Here's how the part is built. I have some questions about the finished solid (model axes, mm). Face numbers are marked on the shaded views. A direction names the side the tool comes from. Give positions to 0.01 mm unless a question says otherwise; leave off trailing zeros. Order: outer loops, then holes, each group sorted by start corner. A loop starts at its lowest first (then second) coordinate and runs counter-clockwise, first axis right, second up. Notation, with made-up numbers: M 29,66.25 L 35,66.25 A13 ccw 35,91.25 Z; hole C -21.75,8 d1. An arc over 180 degrees is marked long. One line per item, written item: value. Start each with the question number.
from build123d import *

# Parameters (mm, degrees)
F0_W     = 38.1
F0_H     = 50.8
F1_DEPTH = 12.7
F2_R     = 1.65
F2_R_2   = 3.5
F3_DEPTH = 12.701
F4_W     = 10
F4_H     = 5
F5_DEPTH = 50.801


with BuildPart() as f1:
    # F0 (on Top) → F1 (new body)
    with BuildSketch(Plane.XY):
        with Locations((19.05, 25.4)):
            Rectangle(F0_W, F0_H)
    extrude(amount=F1_DEPTH)

    # F2 (on face) → F3 (cut, through all)
    with BuildSketch(Plane.XY.offset(12.7)):
        with Locations((8.25, 5)):
            Circle(F2_R)
        with Locations((29.85, 5)):
            Circle(F2_R)
        with Locations((8.25, 25.35)):
            Circle(F2_R)
        with Locations((19.05, 43.5)):
            Circle(F2_R_2)
    extrude(amount=-F3_DEPTH, mode=Mode.SUBTRACT)

    # F4 (on face) → F5 (cut, through all)
    with BuildSketch(Plane.XZ):
        with Locations((18.962298, 2.5)):
            Rectangle(F4_W, F4_H)
    extrude(amount=-F5_DEPTH, mode=Mode.SUBTRACT)


solid = f1.part
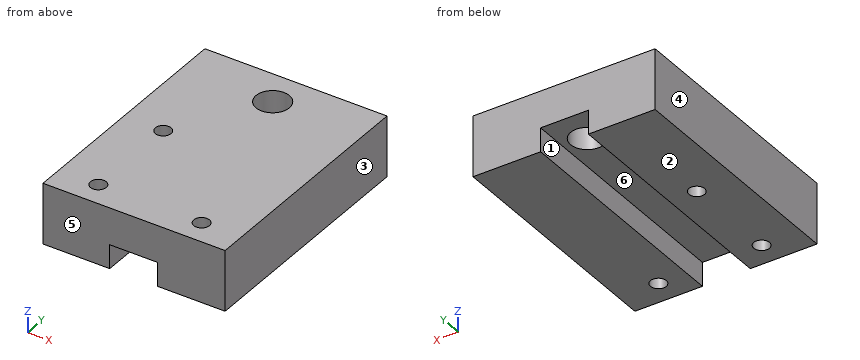
Item 1: Will these pins go through, and if not, where does the flat tip stop? P1, Ø8, axis at x = 19.5, y = 32, coming from the -Z side; P2, Ø2, axis at x = 8.25, y = 25.35, coming from the +Z side.
Item 2: I want a section at D-D on x = 19.05. Write out the boundary of the cut face in (y, z), plus the area to 3 significant figures.
Item 3: I want a section at C-C on y = 43.5. Write out the boundary of the cut face in (x, z).
Item 4: For the marked faces 5 and 6, which set-ups out of +Z, -Z, +X, -X, +Y, -Y let a thin tool reach every point of the face, with its end or its side?
Item 5: We'd pull the mould along X, two halves only. Please class the marked faces 1, 2, 3 and 4: +X half, -X half, draft (parallel to the pull), parting line (faces both ways), or undercut.
Item 6: Please list where these lines run through material, in increasing order: probe 1 along Y at (x, z) = (8.25, 8.5); probe 2 along Y at (x, z) = (19.05, 10); probe 3 along X at (y, z) = (20, 2.75). Write a range as [from, to].
Item 7: I want a section at A-A on z = 4. Write out the boundary of the cut face in (x, y), plus the area to 3 significant figures.
Item 8: I want a section at B-B on x = 8.25. Write out the boundary of the cut face in (y, z), plus the area to 3 significant figures.
Answer below:
1. P1: stops at z = 5
1. P2: passes through
2. outline: M 0,5 L 40,5 L 40,12.7 L 0,12.7 Z; M 47,5 L 50.8,5 L 50.8,12.7 L 47,12.7 Z
2. area: 337 mm²
3. outline: M 0,0 L 13.96,0 L 13.96,5 L 15.55,5 L 15.55,12.7 L 0,12.7 Z; M 22.55,5 L 23.96,5 L 23.96,0 L 38.1,0 L 38.1,12.7 L 22.55,12.7 Z
4. face 5: +Z, -Z, +X, -X, -Y
4. face 6: -Z, +Y, -Y
5. face 1: undercut
5. face 2: draft
5. face 3: +X half
5. face 4: -X half
6. probe 1: y = [0, 3.35], [6.65, 23.7], [27, 50.8]
6. probe 2: y = [0, 40], [47, 50.8]
6. probe 3: x = [0, 13.96], [23.96, 38.1]
7. outline: M 0,0 L 13.96,0 L 13.96,50.8 L 0,50.8 Z; M 23.96,0 L 38.1,0 L 38.1,50.8 L 23.96,50.8 Z; hole C 8.25,5 d3.3; hole C 8.25,25.35 d3.3; hole C 29.85,5 d3.3
7. area: 1,400 mm²
8. outline: M 0,0 L 3.35,0 L 3.35,12.7 L 0,12.7 Z; M 6.65,0 L 23.7,0 L 23.7,12.7 L 6.65,12.7 Z; M 27,0 L 50.8,0 L 50.8,12.7 L 27,12.7 Z
8. area: 561 mm²
